Geometry check sheet. Reference: the model listing, model coordinates, mm. A direction names the side the tool comes from. Coordinates: 2 decimals unless noted, no trailing zeros. Write each loop counter-clockwise with the first axis right and the second up, starting at its lowest first coordinate (ties: lowest second). Pieces come first, ordered by that corner, then holes. Notation, with made-up numbers: (50, 54.5) -> (87, 54.5) arc R12 ccw to (87, 63.5) -> close; hole circle Ø1 at (66.5, -1). An arc over 180 degrees is marked (long way). Use a Markdown table: item, result.
```python
from build123d import *

# Parameters (mm, degrees)
SKETCH1_R           = 3
BOSS_EXTRUDE1_DEPTH = 20
SKETCH4_W           = 7
SKETCH4_H           = 13.6
CUT_EXTRUDE3_DEPTH  = 17
CUT_EXTRUDE4_REACH  = 34
SKETCH5_R           = 4.5
SKETCH7_W           = 15
SKETCH7_H           = 20
CUT_EXTRUDE5_DEPTH  = 10.5
CUT_EXTRUDE6_START  = -2.5
CUT_EXTRUDE6_DEPTH  = 15
FILLET1_R           = 0.1


with BuildPart() as part:
    # Sketch1 → Boss-Extrude1 (new body)
    with BuildSketch(Plane(origin=(0, 0, 0), x_dir=(1, 0, 0), z_dir=(0, 1, 0))):
        with BuildLine():
            Line((-11, -10), (11, -10))
            Line((11, -10), (11, 10))
            Line((11, 10), (-11, 10))
            ThreePointArc((-11, 10), (-21, 0), (-11, -10))
        make_face()
        with Locations((-11, 0)):
            Circle(SKETCH1_R, mode=Mode.SUBTRACT)
    extrude(amount=BOSS_EXTRUDE1_DEPTH)

    # Sketch4 → Cut-Extrude3 (cut)
    with BuildSketch(Plane(origin=(0, 0, -10), x_dir=(-1, 0, 0), z_dir=(0, 0, -1))):
        with Locations((-5, 10)):
            Rectangle(SKETCH4_W, SKETCH4_H)
    extrude(amount=-CUT_EXTRUDE3_DEPTH, mode=Mode.SUBTRACT)

    # Sketch5 → Cut-Extrude4 (cut, up to next)
    with BuildSketch(Plane(origin=(11, 0, 0), x_dir=(0, 0, -1), z_dir=(1, 0, 0)), mode=Mode.PRIVATE) as cut_extrude4_sk1:
        with Locations((0, 10)):
            Circle(SKETCH5_R)
    cut_extrude4_tool1 = extrude(cut_extrude4_sk1.sketch, amount=-CUT_EXTRUDE4_REACH, mode=Mode.PRIVATE) & part.part
    add(cut_extrude4_tool1.solids().sort_by_distance((11, 10, 0))[0], mode=Mode.SUBTRACT)

    # Sketch7 → Cut-Extrude5 (cut, symmetric)
    with BuildSketch(Plane(origin=(-11, 0, 0), x_dir=(0, -1, 0), z_dir=(1, 0, 0))):
        with Locations((-10, 0)):
            Rectangle(SKETCH7_W, SKETCH7_H)
    extrude(amount=CUT_EXTRUDE5_DEPTH, both=True, mode=Mode.SUBTRACT)

    # Sketch8 → Cut-Extrude6 (cut)
    with BuildSketch(Plane.XZ.offset(CUT_EXTRUDE6_START)):
        Polygon((3.215058798, -10), (-0.5, -4.410536459), (-0.5, -10), align=None)
    extrude(amount=-CUT_EXTRUDE6_DEPTH, mode=Mode.SUBTRACT)

    # Fillet1
    fillet1_edges = [part.edges().sort_by_distance(p)[0] for p in [
        (1.5, 10, -7.419621291),
    ]]
    fillet(fillet1_edges, radius=FILLET1_R)


solid = part.part
```
Item 1: Thickness scan on L1, parallel to Y at x = 4, z = -3.75; L2, parallel to Z at x = -11, y = 18.7; L3, parallel to Y at x = -9, z = 6. Record the ranges inside material, lowest first. Write a range as [from, to].
Answer block:
| item | result |
|---|---|
| L1 | y = [0, 3.2], [16.8, 20] |
| L2 | z = [-10, -3], [3, 10] |
| L3 | y = [0, 2.5], [17.5, 20] |
Item 2: Section check D-D on x = 7.5. Record the boundary of the cut face in (y, z), then the cut area to 3 significant figures.
Answer block:
| item | result |
|---|---|
| outline | (0, -10) -> (3.2, -10) -> (3.2, 7) -> (16.8, 7) -> (16.8, -10) -> (20, -10) -> (20, 10) -> (0, 10) -> close |
| area | 169 mm^2 |
Item 3: Mould release check, pull along X, two halves, no side actions. Record for faces 1 (the flat face through (11, 5, 0)), 2 (the cylindrical face through (-13.4, 18.7, 1.8)), 3 (the cylindrical face through (9.77, 14.46, 0.59)): +X half, -X half, draft (parallel to the pull), parting line (faces both ways), or undercut.
Answer block:
| item | result |
|---|---|
| face 1 | +X half |
| face 2 | undercut |
| face 3 | draft |
Item 4: Tool access check on faces 4 (the flat face through (5, 16.8, -2)), 5 (the flat face through (0.145, 9.895, -5.381)), 6 (the flat face through (-0.5, 10, 3)). Record the directions out of +Z, -Z, +X, -X, +Y, -Y that give a thin tool (end or side, any length) a straight path to the whole face; none if there is none.
Answer block:
| item | result |
|---|---|
| face 4 | -Z |
| face 5 | -Z, -X |
| face 6 | +Z, -Z, -X |
Item 5: Section check C-C on y = 11. Record the boundary of the cut face in (x, z), then the cut area to 3 significant figures.
Answer block:
| item | result |
|---|---|
| outline | (-0.5, -4.41) -> (1.32, -7.14) arc R0.1 ccw to (1.5, -7.09) -> (1.5, 7) -> (8.5, 7) -> (8.5, 4.39) -> (11, 4.39) -> (11, 10) -> (-0.5, 10) -> close; (8.5, -10) -> (11, -10) -> (11, -4.39) -> (8.5, -4.39) -> close |
| area | 80.9 mm^2 |
Item 6: Section check B-B on x = -5. Record the boundary of the cut face in (y, z).
Answer block:
| item | result |
|---|---|
| outline | (0, -10) -> (2.5, -10) -> (2.5, 10) -> (0, 10) -> close; (17.5, -10) -> (20, -10) -> (20, 10) -> (17.5, 10) -> close |
Item 7: Section check A-A on z = 0. Record the boundary of the cut face in (x, y).
Answer block:
| item | result |
|---|---|
| outline | (-21, 0) -> (-14, 0) -> (-14, 2.5) -> (-21, 2.5) -> close; (-21, 17.5) -> (-14, 17.5) -> (-14, 20) -> (-21, 20) -> close; (-8, 0) -> (11, 0) -> (11, 5.5) -> (8.5, 5.5) -> (8.5, 3.2) -> (1.5, 3.2) -> (1.5, 16.8) -> (8.5, 16.8) -> (8.5, 14.5) -> (11, 14.5) -> (11, 20) -> (-8, 20) -> (-8, 17.5) -> (-0.5, 17.5) -> (-0.5, 2.5) -> (-8, 2.5) -> close |
Item 8: Depth check by flat-ended pin: P1, Ø11.5, axis at y = 11, z = 0, coming from the -X side; P2, Ø4, axis at y = 9.5, z = 2, coming from the +X side; P3, Ø7.5, axis at x = 3.5, y = 7.5, coming from the -Z side. Enter the tip coordinate at first touch or a pass-through.
Answer block:
| item | result |
|---|---|
| P1 | stops at x = -0.5 |
| P2 | stops at x = 1.5 |
| P3 | stops at z = -7.19 |
